```python
from build123d import *

# Parameters (mm, degrees)
F0_W     = 711.2
F0_H     = 50.8
F1_DEPTH = 50.8
F3_DEPTH = 50.8
F5_DEPTH = 50.8


with BuildPart() as f1:
    # F0 (on Top) → F1 (new body)
    with BuildSketch(Plane.XY):
        Rectangle(F0_W, F0_H)
    extrude(amount=F1_DEPTH)

    # F2 (on face) → F3 (cut)
    with BuildSketch(Plane.XZ.offset(25.4)):
        Polygon((-292.1, 33.02), (-317.5, 33.02), (-317.5, 25.4), (-317.5, 17.78), (-292.1, 17.78), align=None)
    extrude(amount=-F3_DEPTH, mode=Mode.SUBTRACT)

    # F4 (on face) → F5 (cut)
    with BuildSketch(Plane.XZ.offset(25.4)):
        Polygon((317.5, 25.4), (317.5, 33.02), (292.1, 33.02), (292.1, 17.78), (317.5, 17.78), align=None)
    extrude(amount=-F5_DEPTH, mode=Mode.SUBTRACT)


solid = f1.part
```
Model file for the job. Use its own axes, mm. A direction names the side the tool comes from. Round coordinates to 2 decimals unless told otherwise and drop trailing zeros. Order: outer loops, then holes, each group sorted by start corner. A loop starts at its lowest first (then second) coordinate and runs counter-clockwise, first axis right, second up. Notation, with made-up numbers: M 29,11 L 65,11 A24 ccw 65,35 Z; hole C 49.5,-31 d1. An arc over 180 degrees is marked long. Use CSV: the item, a comma, the result in double quotes.
Item 1: Pull direction Z, two halves, no side cores. Call faces 3 (the face through (355.6, 0, 25)), 4 (the face through (-5, 0, 0)), 5 (the face through (-305, 0, 17.78)): released by +Z, released by -Z, zero draft, split by the parting line, or undercut.
Worked answers:
face 3,"zero draft"
face 4,"released by -Z"
face 5,"undercut"
Item 2: Pin check, flat tip, straight feed: pin 1 (12.5 mm diameter, centred on x = -304.5, y = 1, fed in from -Z). Stop position of the tip, or through.
Worked answers:
pin 1,"z = 0"
Item 3: Which spindle directions (+Z, -Z, +X, -X, +Y, -Y) get a long thin tool onto all of the face, cutting with end or side? Do faces 1 (the face through (-5, 25.4, 25)), 2 (the face through (-305, 0, 33.02)). Say none if no direction does.
Worked answers:
face 1,"+Z, -Z, +X, -X, +Y"
face 2,"+Y, -Y"
Item 4: Probe probe 1 along X at (y, z) = (-5.5, 19.5). List the from-to ranges inside material, lowest first.
Worked answers:
probe 1,"-355.6 to -317.5, -292.1 to 292.1, 317.5 to 355.6"
Item 5: Saw through at A-A (y = -1). List the corners of the cut face in (x, z).
Worked answers:
outline,"M -355.6,0 L 355.6,0 L 355.6,50.8 L -355.6,50.8 Z; hole M -317.5,17.78 L -292.1,17.78 L -292.1,33.02 L -317.5,33.02 Z; hole M 292.1,17.78 L 317.5,17.78 L 317.5,33.02 L 292.1,33.02 Z"
